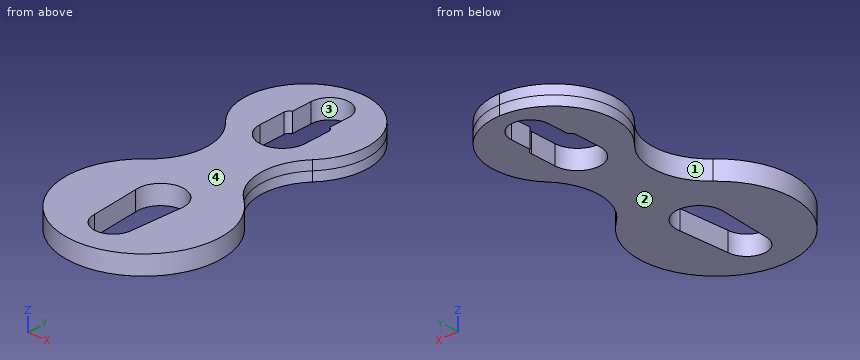
from build123d import *

# Parameters (mm, degrees)
BOSS_EXTRUDE1_DEPTH = 5


with BuildPart() as part:
    # Sketch1 → Boss-Extrude1 (new, symmetric)
    # profile 1 of 2: a face of its own
    with BuildSketch(Plane.XY):
        with BuildLine():
            ThreePointArc((23.298809999, 74.064516129), (29.376312637, 108.689848536), (1.88e-07, 128))
            ThreePointArc((1.88e-07, 128), (-29.376312562, 108.689848709), (-23.298809999, 74.064516129))
            ThreePointArc((-23.298809999, 74.064516129), (-15.190736019, 51.78096855), (-25.79511107, 30.571428571))
            ThreePointArc((-25.79511107, 30.571428571), (0, -40), (25.79511107, 30.571428571))
            ThreePointArc((25.79511107, 30.571428571), (15.190736019, 51.78096855), (23.298809999, 74.064516129))
        make_face()
        with BuildLine():
            ThreePointArc((-11.878172589, 8.294416244), (-11.969504398, 9.1450354), (-12, 10))
            ThreePointArc((-12, 10), (0, 22), (12, 10))
            ThreePointArc((12, 10), (11.969504398, 9.1450354), (11.878172589, 8.294416244))
            Line((11.878172589, 8.294416244), (10, -18))
            ThreePointArc((10, -18), (0, -28), (-10, -18))
            Line((-10, -18), (-11.878172589, 8.294416244))
        make_face(mode=Mode.SUBTRACT)
        with BuildLine():
            ThreePointArc((22, 82), (0, 60), (-22, 82))
            Line((-22, 82), (-22, 106))
            ThreePointArc((-22, 106), (-15.55634912, 121.556349253), (1.88e-07, 128))
            ThreePointArc((1.88e-07, 128), (15.556349253, 121.55634912), (22, 106))
            Line((22, 106), (22, 82))
        make_face(mode=Mode.SUBTRACT)
    # profile 2 of 2: a face of its own
    with BuildSketch(Plane.XY):
        with BuildLine():
            Line((22, 82), (22, 106))
            ThreePointArc((22, 106), (0, 128), (-22, 106))
            Line((-22, 106), (-22, 82))
            ThreePointArc((-22, 82), (0, 60), (22, 82))
        make_face()
        with BuildLine():
            Line((10, 110), (10, 98.828427125))
            ThreePointArc((10, 98.828427125), (11.449489743, 97.732050808), (12, 96))
            Line((12, 96), (12, 82))
            ThreePointArc((12, 82), (0, 70), (-12, 82))
            Line((-12, 82), (-12, 96))
            ThreePointArc((-12, 96), (-11.449489743, 97.732050808), (-10, 98.828427125))
            Line((-10, 98.828427125), (-10, 110))
            ThreePointArc((-10, 110), (0, 120), (10, 110))
        make_face(mode=Mode.SUBTRACT)
    extrude(amount=BOSS_EXTRUDE1_DEPTH, both=True)


solid = part.part
The model under review builds one solid part; all positions refer to its coordinate system, in mm. Face numbers are marked on the shaded views. A direction names the side the tool comes from. Round coordinates to 2 decimals unless told otherwise and drop trailing zeros. Loops run counter-clockwise (first coordinate to the right, second up) from the corner with the lowest first, then second, coordinate; pieces in that order, holes last. Notation, with made-up numbers: M 67,46 L 76,46 A21 ccw 76,83 Z; hole C 84,50 d7. An arc over 180 degrees is marked long. Answer as CSV lines item,"result". Start each with the question number.
Item 1: Consider section B-B (z = 2). Write out the cut boundary in (x, y).
Item 2: Wall thickness on line 1 (X direction, y = -27, z = 2); line 2 (X direction, y = 10, z = 3.25); line 3 (Y direction, x = 3, z = -0.75): over which ranges is each line inside the solid? List them lowest first. Write a range as [from, to].
Item 3: Consider section D-D (y = 48). Write out the cut boundary in (x, z).
Item 4: For the marked faces 3 and 4, list the 3-axis set-ups (+Z, -Z, +X, -X, +Y, -Y) from which the entire face can be reached by the end or side of a thin tool; tool diameter is ignored.
Item 5: Consider section A-A (y = 89). Write out the cut boundary in (x, z), then the cut area to 4 significant figures.
Item 6: Consider section C-C (y = 0). Write out the cut boundary in (x, z), then the cut area to 3 significant figures.
Item 7: Insertion check: P1, Ø1.5, axis at y = 92.5, z = 1, coming from the +X side; P2, Ø5, axis at y = 87.5, z = 2, coming from the -X side; P3, Ø6, axis at y = 63.5, z = 2, coming from the +X side. Each pin has a flat end and moves straight along its axis. Give the tip position at first contact, or say it passes through.
Item 8: Mouldability with a two-part tool opening along Y and no side actions: class the marked faces 1 and 2 as released by +Y, released by -Y, zero draft, split by the parting line, or undercut.
Answer:
1,outline,"M -25.8,30.57 A40 ccw long 25.8,30.57 A30 cw 23.3,74.06 A32 ccw long -23.3,74.06 A30 cw Z; hole M -12,82 A12 ccw 12,82 L 12,96 A3 ccw 10,98.83 L 10,110 A10 ccw -10,110 L -10,98.83 A3 ccw -12,96 Z; hole M -11.88,8.29 L -10,-18 A10 ccw 10,-18 L 11.88,8.29 A12 ccw long Z"
2,line 1,"x = [-29.51, -4.36], [4.36, 29.51]"
2,line 2,"x = [-38.73, -12], [12, 38.73]"
2,line 3,"y = [-39.89, -27.54], [21.62, 70.38], [119.54, 127.86]"
3,outline,"M -15.65,-5 L 15.65,-5 L 15.65,5 L -15.65,5 Z"
4,face 3,"+Z, -Z"
4,face 4,"+Z, +X, -X, +Y, -Y"
5,outline,"M -31.22,-5 L -12,-5 L -12,5 L -31.22,5 Z; M 12,-5 L 31.22,-5 L 31.22,5 L 12,5 Z"
5,area,"384.5 mm^2"
6,outline,"M -40,-5 L -11.29,-5 L -11.29,5 L -40,5 Z; M 11.29,-5 L 40,-5 L 40,5 L 11.29,5 Z"
6,area,"574 mm^2"
7,P1,"stops at x = 31.88"
7,P2,"stops at x = -31.43"
7,P3,"stops at x = 18.1"
8,face 1,"undercut"
8,face 2,"zero draft"
